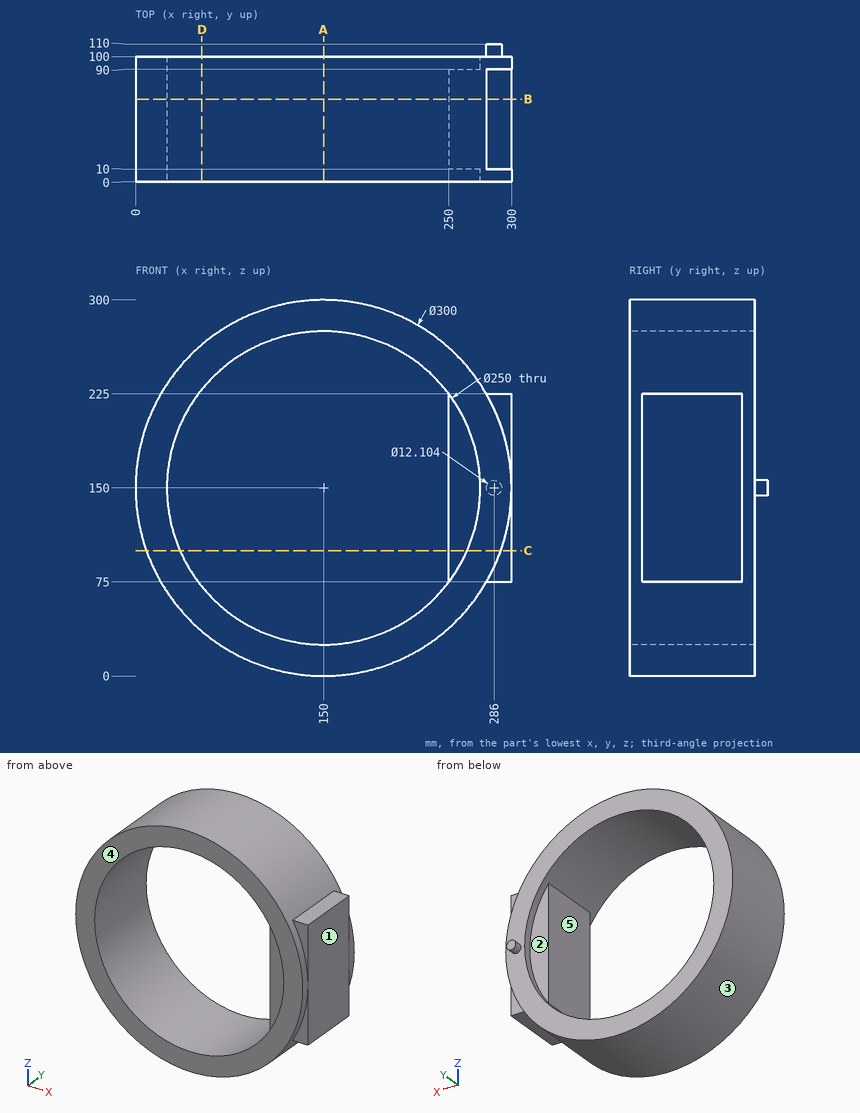
Part print with two shaded views. Sizes in mm from the minimum x, y, z corner. A direction names the side the tool comes from. Coordinates: 2 decimals unless noted, no trailing zeros. Loops run counter-clockwise (first coordinate to the right, second up) from the corner with the lowest first, then second, coordinate; pieces in that order, holes last. Notation, with made-up numbers: (66.25, -1) -> (116.25, -1) arc R29 ccw to (116.25, 29) -> close; hole circle Ø11 at (-28, -37). An arc over 180 degrees is marked (long way). Answer as a JSON object with one key per item and string values.
Q1. Probe probe 1 along Z at (x, y) = (150, 56); probe 2 along X at (y, z) = (67.5, 238) (3 decimals); probe 3 along X at (y, z) = (72, 83) (3 decimals). List the from-to ranges inside material, lowest first.
Report:
{"probe 1": "z = 0 to 25, 275 to 300", "probe 2": "x = 28.526 to 61.225, 238.775 to 271.474", "probe 3": "x = 15.795 to 44.473, 250 to 300"}
Q2. Flat gauge pins, fed straight in: P1, Ø1.5, axis at x = 42.5, y = 27.5, coming from the +Z side; P2, Ø8, axis at x = 268, y = 68, coming from the +Z side; P3, Ø6, axis at x = 289.5, z = 117.5, coming from the +Y side; P4, Ø4, axis at x = 208, z = 43.5, coming from the +Y side. Where does each tip first touch, or does it go through?
Report:
{"P1": "stops at z = 255.38", "P2": "stops at z = 247.49", "P3": "stops at y = 100", "P4": "passes through"}
Q3. 3-axis set-ups, long thin cutter, end or side, ignore diameter. For the marked faces 4 and 5: which of +Z, -Z, +X, -X, +Y, -Y reach the whole face in a straight line?
Report:
{"face 4": "+Z, -Z, +X, -X, -Y", "face 5": "+Y, -Y"}
Q4. Cut at C-C (z = 100). List the corners of the cut face in (x, y), and give its area (3 significant figures).
Report:
{"outline": "(8.58, 0) -> (35.44, 0) -> (35.44, 100) -> (8.58, 100) -> close; (250, 10) -> (264.56, 10) -> (264.56, 0) -> (291.42, 0) -> (291.42, 10) -> (300, 10) -> (300, 90) -> (291.42, 90) -> (291.42, 100) -> (264.56, 100) -> (264.56, 90) -> (250, 90) -> close", "area": "7,220 mm2"}
Q5. Pull direction Z, two halves, no side cores. Call the marked faces 1, 2 and 3: released by +Z, released by -Z, zero draft, split by the parting line, or undercut.
Report:
{"face 1": "zero draft", "face 2": "undercut", "face 3": "split by the parting line"}
Q6. Cut at B-B (y = 66). List the corners of the cut face in (x, z), and give its area (3 significant figures).
Report:
{"outline": "(279.9, 75) -> (300, 75) -> (300, 225) -> (279.9, 225) arc R150 ccw (long way) to start; hole (250, 75) -> (250, 225) arc R125 ccw (long way) to start", "area": "25,100 mm2"}
Q7. Cut at A-A (x = 150). List the corners of the cut face in (y, z), and give its area (3 significant figures).
Report:
{"outline": "(0, 0) -> (100, 0) -> (100, 25) -> (0, 25) -> close; (0, 275) -> (100, 275) -> (100, 300) -> (0, 300) -> close", "area": "5,000 mm2"}
Q8. Cut at D-D (x = 53). List the corners of the cut face in (y, z), and give its area (3 significant figures).
Report:
{"outline": "(0, 35.58) -> (100, 35.58) -> (100, 71.16) -> (0, 71.16) -> close; (0, 228.84) -> (100, 228.84) -> (100, 264.42) -> (0, 264.42) -> close", "area": "7,110 mm2"}
